Geometry check sheet. Reference: the model listing, model coordinates, mm. A direction names the side the tool comes from. Give positions to 0.01 mm unless a question says otherwise; leave off trailing zeros. Loops run counter-clockwise (first coordinate to the right, second up) from the corner with the lowest first, then second, coordinate; pieces in that order, holes last. Notation, with made-up numbers: (-10.75, 17.5) - (16.25, 17.5) arc R28 ccw to (16.25, 50.5) - close; hole circle Ø1 at (40, 50.5). An arc over 180 degrees is marked (long way). Use a Markdown table: item, result. Add a question column.
1. Draft check along X on faces 3 (the flat face through (-425.45, 0, 2)), 4 (the flat face through (-430, 25.4, 2)), 5 (the cylindrical face through (-459.7, 19.3, 1.6)). Enter one of: pulls with the +X half, pulls with the -X half, needs draft (parallel to the pull), parting line crosses it, or undercut.
2. Cross-section at C-C on z = 2.55. Count the separate pieces of the cut face and the enclosed holes in it, and give its area (3 significant figures).
3. Set-up check for faces 1 (the cylindrical face through (-495.87, 0.09, 1.57)), 2 (the flat face through (-430, -25.4, 2)): record each of +Z, -Z, +X, -X, +Y, -Y from which the full face is reachable in a straight line by a thin tool's end or side.
4. Cross-section at D-D on x = -495. Enter the section's corners in (y, z) (3 decimals).
5. Cross-section at B-B on y = -12.7. Enter the section's corners in (x, z) (3 decimals).
6. Material ranges on L1, parallel to Y at x = -431.8, z = 1.75; L2, parallel to Y at x = -469.5, z = 2.95; L3, parallel to X at y = 21, z = 0.4, recorded low to high.
7. Cross-section at A-A on x = -469.9. Enter the section's corners in (y, z) (3 decimals), and give its area (3 significant figures).
8. Depth check by flat-ended pin: P1, Ø6, axis at x = -431.8, y = 12.7, coming from the -Z side; P2, Ø1.6, axis at x = -429, z = 1.5, coming from the -Y side. Enter the tip coordinate at first touch or a pass-through.
from build123d import *

# Parameters (mm, degrees)
SKETCH2_R           = 15.875
SKETCH2_R_2         = 2.159
SKETCH2_R_3         = 2.54
BOSS_EXTRUDE1_DEPTH = 3.175
FILLET1_R           = 2.54
SKETCH3_OUTSIDE_W   = 172.398
SKETCH3_OUTSIDE_H   = 96.198
SKETCH3_OUTSIDE_W_2 = 82.55
SKETCH3_OUTSIDE_H_2 = 74.066797773
CUT_EXTRUDE1_DEPTH  = 510.001122911
FILLET2_R           = 2.54


with BuildPart() as part:
    # Sketch2 → Boss-Extrude1 (new body)
    with BuildSketch(Plane.XY):
        Polygon((-508, 25.4), (-481.80625, 31.75), (-457.99375, 31.75), (-431.8, 25.4), (-368.3, 25.4), (-368.3, -25.4), (-431.8, -25.4), (-457.99375, -31.75), (-481.80625, -31.75), (-508, -25.4), align=None)
        with Locations((-469.9, 0)):
            Circle(SKETCH2_R, mode=Mode.SUBTRACT)
        with Locations((-457.99375, 20.622229928)):
            Circle(SKETCH2_R_2, mode=Mode.SUBTRACT)
        with Locations((-481.80625, 20.622229928)):
            Circle(SKETCH2_R_2, mode=Mode.SUBTRACT)
        with Locations((-493.7125, 0)):
            Circle(SKETCH2_R_2, mode=Mode.SUBTRACT)
        with Locations((-481.80625, -20.622229928)):
            Circle(SKETCH2_R_2, mode=Mode.SUBTRACT)
        with Locations((-457.99375, -20.622229928)):
            Circle(SKETCH2_R_2, mode=Mode.SUBTRACT)
        with Locations((-446.0875, 0)):
            Circle(SKETCH2_R_2, mode=Mode.SUBTRACT)
        with Locations((-495.3, 12.7)):
            Circle(SKETCH2_R_3, mode=Mode.SUBTRACT)
        with Locations((-495.3, -12.7)):
            Circle(SKETCH2_R_3, mode=Mode.SUBTRACT)
        with Locations((-444.5, -12.7)):
            Circle(SKETCH2_R_3, mode=Mode.SUBTRACT)
        with Locations((-431.8, -12.7)):
            Circle(SKETCH2_R_3, mode=Mode.SUBTRACT)
        with Locations((-419.1, -12.7)):
            Circle(SKETCH2_R_3, mode=Mode.SUBTRACT)
        with Locations((-419.1, 0)):
            Circle(SKETCH2_R_3, mode=Mode.SUBTRACT)
        with Locations((-431.8, 0)):
            Circle(SKETCH2_R_3, mode=Mode.SUBTRACT)
        with Locations((-431.8, 12.7)):
            Circle(SKETCH2_R_3, mode=Mode.SUBTRACT)
        with Locations((-419.1, 12.7)):
            Circle(SKETCH2_R_3, mode=Mode.SUBTRACT)
        with Locations((-444.5, 12.7)):
            Circle(SKETCH2_R_3, mode=Mode.SUBTRACT)
        with Locations((-406.4, 12.7)):
            Circle(SKETCH2_R_3, mode=Mode.SUBTRACT)
        with Locations((-406.4, 0)):
            Circle(SKETCH2_R_3, mode=Mode.SUBTRACT)
        with Locations((-406.4, -12.7)):
            Circle(SKETCH2_R_3, mode=Mode.SUBTRACT)
        with Locations((-393.7, 12.7)):
            Circle(SKETCH2_R_3, mode=Mode.SUBTRACT)
        with Locations((-393.7, 0)):
            Circle(SKETCH2_R_3, mode=Mode.SUBTRACT)
        with Locations((-393.7, -12.7)):
            Circle(SKETCH2_R_3, mode=Mode.SUBTRACT)
        with Locations((-381, 12.7)):
            Circle(SKETCH2_R_3, mode=Mode.SUBTRACT)
        with Locations((-381, 0)):
            Circle(SKETCH2_R_3, mode=Mode.SUBTRACT)
        with Locations((-381, -12.7)):
            Circle(SKETCH2_R_3, mode=Mode.SUBTRACT)
    extrude(amount=BOSS_EXTRUDE1_DEPTH)

    # Fillet1
    fillet1_edges = [part.edges().sort_by_distance(p)[0] for p in [
        (-508, 25.4, 1.5875),
        (-481.80625, 31.75, 1.5875),
        (-457.99375, 31.75, 1.5875),
        (-431.8, 25.4, 1.5875),
        (-368.3, 25.4, 1.5875),
        (-368.3, -25.4, 1.5875),
        (-431.8, -25.4, 1.5875),
        (-457.99375, -31.75, 1.5875),
        (-481.80625, -31.75, 1.5875),
        (-508, -25.4, 1.5875),
    ]]
    fillet(fillet1_edges, radius=FILLET1_R)

    # Sketch3 outside → Cut-Extrude1 (cut, through all)
    with BuildSketch(Plane.XY.offset(3.175)):
        with Locations((-438.15, 0)):
            Rectangle(SKETCH3_OUTSIDE_W, SKETCH3_OUTSIDE_H)
        with Locations((-466.725, 2.505642685)):
            Rectangle(SKETCH3_OUTSIDE_W_2, SKETCH3_OUTSIDE_H_2, mode=Mode.SUBTRACT)
    extrude(amount=-CUT_EXTRUDE1_DEPTH, mode=Mode.SUBTRACT)

    # Fillet2
    fillet2_edges = [part.edges().sort_by_distance(p)[0] for p in [
        (-425.45, 25.4, 1.5875),
        (-425.45, -25.4, 1.5875),
    ]]
    fillet(fillet2_edges, radius=FILLET2_R)


solid = part.part
Values found:
| question | item | result |
|---|---|---|
| 1 | face 3 | pulls with the +X half |
| 1 | face 4 | needs draft |
| 1 | face 5 | undercut |
| 2 | separate pieces | 1 |
| 2 | enclosed holes | 14 |
| 2 | area | 3,800 mm2 |
| 3 | face 1 | +Z, -Z |
| 3 | face 2 | +Z, -Z, +X, -Y |
| 4 | outline | (-28.552, 0) - (-15.222, 0) - (-15.222, 3.175) - (-28.552, 3.175) - close; (-10.178, 0) - (-1.733, 0) - (-1.733, 3.175) - (-10.178, 3.175) - close; (1.733, 0) - (10.178, 0) - (10.178, 3.175) - (1.733, 3.175) - close; (15.222, 0) - (28.552, 0) - (28.552, 3.175) - (15.222, 3.175) - close |
| 5 | outline | (-508, 0) - (-497.84, 0) - (-497.84, 3.175) - (-508, 3.175) - close; (-492.76, 0) - (-479.425, 0) - (-479.425, 3.175) - (-492.76, 3.175) - close; (-460.375, 0) - (-447.04, 0) - (-447.04, 3.175) - (-460.375, 3.175) - close; (-441.96, 0) - (-434.34, 0) - (-434.34, 3.175) - (-441.96, 3.175) - close; (-429.26, 0) - (-425.45, 0) - (-425.45, 3.175) - (-429.26, 3.175) - close |
| 6 | L1 | y = -25.42 to -15.24, -10.16 to -2.54, 2.54 to 10.16, 15.24 to 25.42 |
| 6 | L2 | y = -31.75 to -15.87, 15.87 to 31.75 |
| 6 | L3 | x = -508 to -483.93, -479.68 to -460.12, -455.87 to -425.45 |
| 7 | outline | (-31.75, 0) - (-15.875, 0) - (-15.875, 3.175) - (-31.75, 3.175) - close; (15.875, 0) - (31.75, 0) - (31.75, 3.175) - (15.875, 3.175) - close |
| 7 | area | 101 mm2 |
| 8 | P1 | stops at z = 0 |
| 8 | P2 | stops at y = -25.4 |
